Source: CAD feature listing. Evaluate the final solid. Frame: model axes, mm. Coordinates: 2 decimals unless noted, no trailing zeros. Write each loop counter-clockwise with the first axis right and the second up, starting at its lowest first coordinate (ties: lowest second). Pieces come first, ordered by that corner, then holes. Notation, with made-up numbers: (-24.75, -39.75) - (-13.75, -39.75) arc R25 ccw to (-13.75, -14.75) - close; hole circle Ø1 at (41.5, -22). An arc over 180 degrees is marked (long way). One line per question, with ' | ' between items.
from build123d import *

# Parameters (mm, degrees)
ESQUISSE1_R        = 5
BOSS_EXTRU_1_DEPTH = 1000
ESQUISSE2_R        = 4
BOSS_EXTRU_2_DEPTH = 20
BOSS_EXTRU_3_START = 20
ESQUISSE3_R        = 4
BOSS_EXTRU_3_DEPTH = 20
D_GAGEMENT_M11_D   = 1.2


with BuildPart() as part:
    # Esquisse1 → Boss.-Extru.1 (new body)
    with BuildSketch(Plane(origin=(0, 0, 0), x_dir=(1, 0, 0), z_dir=(0, 1, 0))):
        with Locations(Location((0, 0, 0), (0, 0, 270))):
            Circle(ESQUISSE1_R)
    extrude(amount=BOSS_EXTRU_1_DEPTH)

    # Esquisse2 → Boss.-Extru.2 (add)
    with BuildSketch(Plane(origin=(0, 1000, 0), x_dir=(1, 0, 0), z_dir=(0, 1, 0))):
        with Locations(Location((0, 0, 0), (0, 0, 270))):
            Circle(ESQUISSE2_R)
    extrude(amount=BOSS_EXTRU_2_DEPTH)

    # Esquisse3 → Boss.-Extru.3 (add)
    with BuildSketch(Plane(origin=(0, 0, 0), x_dir=(-1, 0, 0), z_dir=(0, -1, 0)).offset(BOSS_EXTRU_3_START)):
        with Locations(Location((0, 0, 0), (0, 0, 270))):
            Circle(ESQUISSE3_R)
    extrude(amount=-BOSS_EXTRU_3_DEPTH)

    # Dégagement M11 (through all)
    with Locations(Plane(origin=(5, 520, 0), x_dir=(0, 0, 1), z_dir=(1, 0, 0))):
        with Locations((0, 0)):
            Hole(D_GAGEMENT_M11_D / 2)


solid = part.part
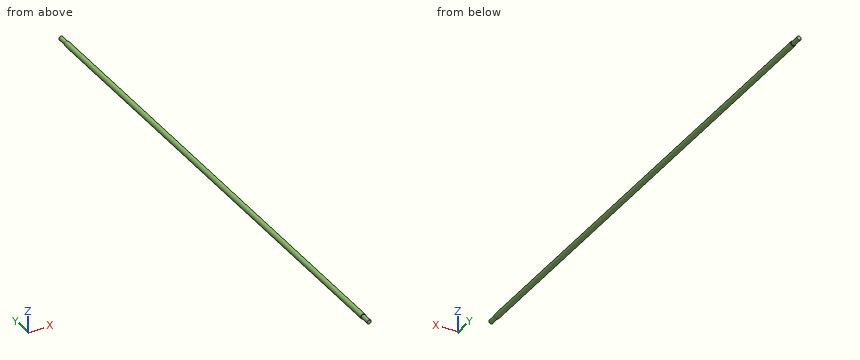
Item 1: Pin query (flat end, axial travel): pin 1 Ø4 at (y, z) = (153.5, 4) entering from +X; pin 2 Ø1 at (y, z) = (520, 0) entering from +X; pin 3 Ø3 at (y, z) = (718, 2.5) entering from +X; pin 4 Ø4 at (x, y) = (3, 474.5) entering from +Z. Return the tip coordinate at first contact, or that it passes through.
Check sheet entries:
pin 1: x = 4.58 | pin 2: through | pin 3: x = 4.9 | pin 4: z = 4.9
Item 2: Cut plane A-A on y = 889. Return loops of the section in (x, z), and give its area (3 significant figures).
Check sheet entries:
outline: circle Ø10 at (0, 0) | area: 78.5 mm²
Item 3: Ray query, line 1 along Y through (x, z) = (2.5, 0); line 2 along Z through (x, y) = (0.75, 520); line 3 along Z through (x, y) = (-1, 835.5). Return the intervals inside material, ascending. Write a range as [from, to].
Check sheet entries:
line 1: [-20, 519.4], [520.6, 1020] | line 2: [-4.94, -0.6], [0.6, 4.94] | line 3: [-4.9, 4.9]
